CAD build for the part. Positions are in the model's coordinates, mm. Face numbers are marked on the shaded views. A direction names the side the tool comes from. Coordinates: 2 decimals unless noted, no trailing zeros. Loops run counter-clockwise (first coordinate to the right, second up) from the corner with the lowest first, then second, coordinate; pieces in that order, holes last. Notation, with made-up numbers: (-38.5, -28.75) -> (7.5, -28.75) arc R24 ccw to (7.5, 8.25) -> close; hole circle Ø8 at (58, 46.5). An arc over 180 degrees is marked (long way). Return JSON: item names as keys, results as strings. Group by question number.
(1) Saw through at C-C on z = 6.5. Write the cut outline in (x, y).
(2) Mould opens along Z. For the marked faces 5, 6 and 7 say: pulls with the +Z half, pulls with the -Z half, needs draft (parallel to the pull), parting line crosses it, or undercut.
(3) Saw through at B-B on y = -0.5. Write the cut outline in (x, z).
(4) Saw through at A-A on x = 2.6. Write the cut outline in (y, z).
(5) Probe L1, parallel to Z at x = -1.7, y = -2.5; L2, parallel to X at y = -0.75, z = 6.5; L3, parallel to Z at x = 0.1, y = 0. List the from-to ranges inside material, lowest first.
(6) Tool access for the marked faces 1, 2, 3 and 4: list every direction of +Z, -Z, +X, -X, +Y, -Y with a clear straight run to the whole face (end or side of a thin tool).
(7) Saw through at D-D on x = 0. Write the cut outline in (y, z).
(8) Flat gauge pins, fed straight in: pin 1 Ø0.8 at (x, z) = (-1, -1.5) entering from -Y; pin 2 Ø1.6 at (x, y) = (-2, 1.5) entering from -Z. Where does each tip first touch, or does it go through?
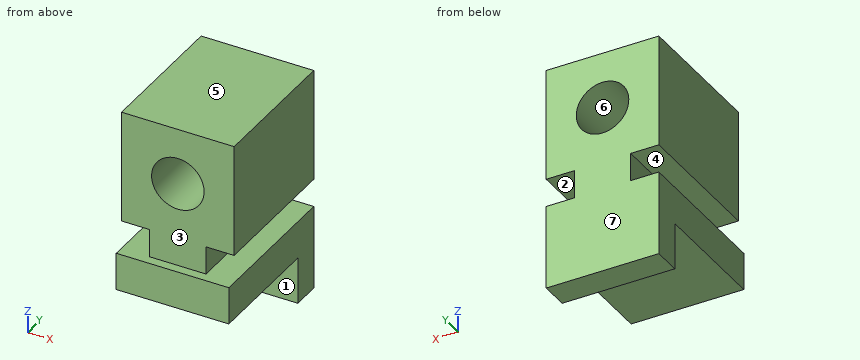
```python
from build123d import *

# Parameters (mm, degrees)
SKETCH3_W           = 6
SKETCH3_H           = 6.5
BOSS_EXTRUDE3_DEPTH = 2
SKETCH4_W           = 3
SKETCH4_H           = 1.5
BOSS_EXTRUDE4_DEPTH = 6
SKETCH5_W           = 6
SKETCH5_H           = 6
SKETCH5_R           = 1.4
BOSS_EXTRUDE5_DEPTH = 6
BOSS_EXTRUDE6_START = 1.5
SKETCH9_R           = 1.4
BOSS_EXTRUDE6_DEPTH = 1.5
SKETCH10_W          = 6
SKETCH10_H          = 1.5
BOSS_EXTRUDE7_DEPTH = 2.5


with BuildPart() as part:
    # Sketch3 → Boss-Extrude3 (new body)
    with BuildSketch(Plane.XY):
        Rectangle(SKETCH3_W, SKETCH3_H)
    extrude(amount=BOSS_EXTRUDE3_DEPTH)

    # Sketch4 → Boss-Extrude4 (add)
    with BuildSketch(Plane(origin=(0, 3.25, 0), x_dir=(1, 0, 0), z_dir=(0, 1, 0))):
        with Locations((0, -2.75)):
            Rectangle(SKETCH4_W, SKETCH4_H)
    extrude(amount=-BOSS_EXTRUDE4_DEPTH)

    # Sketch5 → Boss-Extrude5 (add)
    with BuildSketch(Plane(origin=(0, 3.25, 0), x_dir=(1, 0, 0), z_dir=(0, 1, 0))):
        with Locations((0, -6.5)):
            Rectangle(SKETCH5_W, SKETCH5_H)
        with Locations(Location((0, -6.5, 0), (0, 0, 270))):
            Circle(SKETCH5_R, mode=Mode.SUBTRACT)
    extrude(amount=-BOSS_EXTRUDE5_DEPTH)

    # Sketch9 → Boss-Extrude6 (add)
    with BuildSketch(Plane(origin=(0, 3.25, 0), x_dir=(1, 0, 0), z_dir=(0, 1, 0)).offset(BOSS_EXTRUDE6_START)):
        Polygon((3, -9.5), (-3, -9.5), (-3, -3.5), (-1.5, -3.5), (-1.5, -2), (-3, -2), (-3, 0), (3, 0), (3, -2), (1.5, -2), (1.5, -3.5), (3, -3.5), align=None)
        with Locations(Location((0, -6.5, 0), (0, 0, 270))):
            Circle(SKETCH9_R, mode=Mode.SUBTRACT)
    extrude(amount=-BOSS_EXTRUDE6_DEPTH)

    # Sketch10 → Boss-Extrude7 (add)
    with BuildSketch(Plane(origin=(0, 0, 0), x_dir=(-1, 0, 0), z_dir=(0, 0, -1))):
        with Locations((0, 4)):
            Rectangle(SKETCH10_W, SKETCH10_H)
    extrude(amount=BOSS_EXTRUDE7_DEPTH)


solid = part.part
```
Geometry results:
{
 "1": {"outline": "(-3, -2.75) -> (-1.4, -2.75) -> (-1.4, 4.75) -> (-3, 4.75) -> close; (1.4, -2.75) -> (3, -2.75) -> (3, 4.75) -> (1.4, 4.75) -> close"},
 "2": {"face 5": "pulls with the +Z half", "face 6": "undercut", "face 7": "needs draft"},
 "3": {"outline": "(-3, 0) -> (3, 0) -> (3, 2) -> (1.5, 2) -> (1.5, 3.5) -> (3, 3.5) -> (3, 9.5) -> (-3, 9.5) -> (-3, 3.5) -> (-1.5, 3.5) -> (-1.5, 2) -> (-3, 2) -> close; hole circle Ø2.8 at (0, 6.5)"},
 "4": {"outline": "(-3.25, 0) -> (3.25, 0) -> (3.25, -2.5) -> (4.75, -2.5) -> (4.75, 2) -> (-3.25, 2) -> close; (-2.75, 3.5) -> (4.75, 3.5) -> (4.75, 9.5) -> (-2.75, 9.5) -> close"},
 "5": {"L1": "0 to 2, 3.5 to 9.5", "L2": "-3 to -1.4, 1.4 to 3", "L3": "0 to 5.1, 7.9 to 9.5"},
 "6": {"face 1": "-Z, +X, -X, -Y", "face 2": "+X, +Y, -Y", "face 3": "+Z, +X, -X, -Y", "face 4": "-X, +Y, -Y"},
 "7": {"outline": "(-3.25, 0) -> (3.25, 0) -> (3.25, -2.5) -> (4.75, -2.5) -> (4.75, 5.1) -> (-2.75, 5.1) -> (-2.75, 2) -> (-3.25, 2) -> close; (-2.75, 7.9) -> (4.75, 7.9) -> (4.75, 9.5) -> (-2.75, 9.5) -> close"},
 "8": {"pin 1": "y = 3.25", "pin 2": "z = 0"}
}
